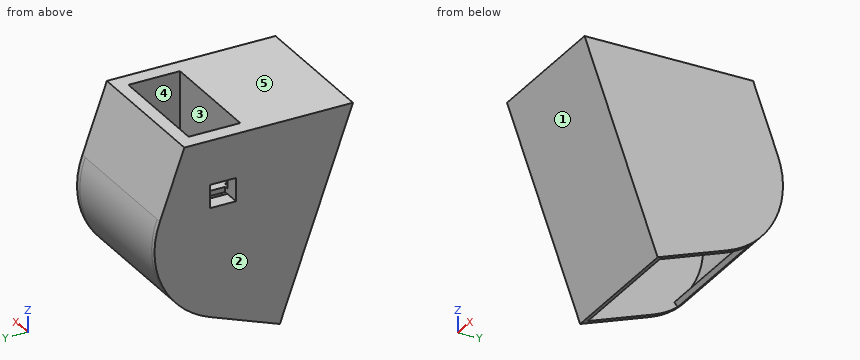
from build123d import *

# Parameters (mm, degrees)
F0_W      = 53.34
F0_H      = 25.4
F0_R      = 1.27
F1_DEPTH  = 2.54
F3_DEPTH  = 53.34
F5_DEPTH  = 7.62
F6_W      = 12.7
F6_H      = 8.89
F7_DEPTH  = 7.62
F8_W      = 12.7
F8_H      = 2.54
F9_DEPTH  = 9.525
F10_W     = 68.58
F10_H     = 41.6090539173
F11_DEPTH = 2.54
F13_REACH = 169.3857709485
F15_DEPTH = 63.5
F17_DEPTH = 2.54
F19_DEPTH = 2.54
F21_DEPTH = 2.54
F22_W     = 63.5
F22_H     = 2.54


with BuildPart() as f1:
    # F0 (on Top) → F1 (new body)
    with BuildSketch(Plane.XY):
        Rectangle(F0_W, F0_H)
        with Locations((-22.86, -8.89)):
            Circle(F0_R, mode=Mode.SUBTRACT)
        with Locations((22.86, -8.89)):
            Circle(F0_R, mode=Mode.SUBTRACT)
        with Locations((-22.86, 8.89)):
            Circle(F0_R, mode=Mode.SUBTRACT)
        with Locations((22.86, 8.89)):
            Circle(F0_R, mode=Mode.SUBTRACT)
    extrude(amount=F1_DEPTH)

    # F2 (on face) → F3 (join, through all)
    with BuildSketch(Plane.YZ.offset(26.67)):
        Polygon((-15.24, -0.447870531), (-9.9437557743, -14.9991819491), (-7.5569365175, -14.130450785), (-12.7, 0), (-12.7, 2.54), (-12.7, 33.02), (-27.4213086776, 33.02), (-26.4968242825, 30.48), (-15.24, 30.48), align=None)
        Polygon((-26.4968242825, 30.48), (-15.24, -0.447870531), (-15.24, 30.48), align=None)
    extrude(amount=-F3_DEPTH)



with BuildPart() as f3:
    # F2 (on face) → F3, piece 2 (new body, through all)
    with BuildSketch(Plane.YZ.offset(26.67)):
        Polygon((12.7, 33.02), (12.7, 30.48), (17.2714728529, 30.48), (28.7046231961, -0.9323224012), (31.0914424529, -0.0635912371), (19.05, 33.02), align=None)
    extrude(amount=-F3_DEPTH)


with BuildPart() as f1_1:
    add(f1.part)

    add(f3.part)  # F5 merges F3
    # F4 (on face) → F5 (join)
    with BuildSketch(Plane.YZ.offset(26.67)):
        Polygon((-27.4213086776, 33.02), (-9.9437557743, -14.9991819491), (31.0914424529, -0.0635912371), (19.05, 33.02), align=None)
    extrude(amount=F5_DEPTH)

    # F6 (on face) → F7 (join)
    with BuildSketch(Plane(origin=(-26.67, 0, 0), x_dir=(0, -1, 0), z_dir=(-1, 0, 0))):
        Polygon((9.9437557743, -14.9991819491), (27.4213086776, 33.02), (-19.05, 33.02), (-31.0914424529, -0.0635912371), align=None)
        with Locations((0, 6.985)):
            Rectangle(F6_W, F6_H, mode=Mode.SUBTRACT)
    extrude(amount=F7_DEPTH)

    # F8 (on face) → F9 (cut)
    with BuildSketch(Plane(origin=(-34.29, 0, 0), x_dir=(0, -1, 0), z_dir=(-1, 0, 0))):
        with Locations((0, 1.27)):
            Rectangle(F8_W, F8_H)
    extrude(amount=-F9_DEPTH, mode=Mode.SUBTRACT)

    # F10 (on face) → F11 (join, through all)
    with BuildSketch(Plane(origin=(0, -13.6012014706, -4.9504324856), x_dir=(1, 0, 0), z_dir=(0, -0.9396926208, -0.3420201433))):
        with Locations((0, -31.4981827789)):
            Rectangle(F10_W, F10_H)
    extrude(amount=-F11_DEPTH)

    f13_end = Plane(origin=(0, -7.2808291762, 33.02), x_dir=(1, 0, 0), z_dir=(0, 0, 1))
    # F12 (on face) → F13 (join, up to a plane its end follows)
    with BuildSketch(Plane(origin=(0, 17.8885802808, -49.1484703875), x_dir=(1, 0, 0), z_dir=(0, 0.3420201433, -0.9396926208))):
        Polygon((31.75, 14.474096284), (34.29, 14.474096284), (34.29, 48.764096284), (-34.29, 48.764096284), (-34.29, 14.474096284), (-31.75, 14.474096284), (-31.75, 46.224096284), (31.75, 46.224096284), align=None)
    f13_long = extrude(amount=-F13_REACH, mode=Mode.PRIVATE)
    add(split(f13_long, bisect_by=f13_end, keep=Keep.BOTTOM, mode=Mode.PRIVATE))

    # F14 (on face) → F15 (join, through all)
    with BuildSketch(Plane(origin=(31.75, 0, 0), x_dir=(0, -1, 0), z_dir=(-1, 0, 0))):
        Polygon((27.4213086775, 33.02), (26.5525775135, 30.6331807432), (60.3402217897, 30.6331807432), (61.2089529537, 33.02), align=None)
    extrude(amount=F15_DEPTH)

    # F16 (on face) → F17 (cut, through all)
    with BuildSketch(Plane(origin=(0, -11.2143822138, -4.0817013215), x_dir=(-1, 0, 0), z_dir=(0, 0.9396926208, 0.3420201433))):
        Polygon((26.67, 4.3436558202), (-26.67, 4.3436558202), (-26.67, -10.6936558203), (-31.75, -10.6936558203), (-31.75, -52.3027097376), (31.75, -52.3027097376), (31.75, -10.6936558203), (26.67, -10.6936558203), align=None)
    extrude(amount=-F17_DEPTH, mode=Mode.SUBTRACT)

    # F18 (on face) → F19 (join)
    with BuildSketch(Plane.YZ.offset(34.29)):
        with BuildLine():
            ThreePointArc((6.6741980668, -53.230171709), (29.9844867323, -31.7454245982), (31.0914424529, -0.0635912371))
            Line((31.0914424529, -0.0635912371), (-7.5569365175, -14.130450785))
            Line((-7.5569365176, -14.130450785), (6.6741980668, -53.230171709))
        make_face()
    extrude(amount=-F19_DEPTH)

    # F20 (on face) → F21 (join)
    with BuildSketch(Plane(origin=(-34.29, 0, 0), x_dir=(0, -1, 0), z_dir=(-1, 0, 0))):
        with BuildLine():
            ThreePointArc((-31.0914424529, -0.0635912371), (-29.9844867323, -31.7454245982), (-6.6741980668, -53.230171709))
            Line((-6.6741980669, -53.230171709), (7.5569365175, -14.130450785))
            Line((7.5569365175, -14.130450785), (-31.0914424529, -0.0635912371))
        make_face()
    extrude(amount=-F21_DEPTH)

    # F24: sweep along a path in F23
    with BuildLine(Plane(origin=(31.75, 0, 0), x_dir=(0, -1, 0), z_dir=(-1, 0, 0))) as f24_path:
        ThreePointArc((-18.5834505022, -46.4695330224), (-32.3206049052, -25.2835298235), (-31.0914424529, -0.0635912371))
    # F22 (on face) → F24 (sweep)
    with BuildSketch(Plane(origin=(0, 3.6574456963, -10.0487494635), x_dir=(1, 0, 0), z_dir=(0, 0.3420201433, -0.9396926208))):
        with Locations((0, -27.9246495586)):
            Rectangle(F22_W, F22_H)
    sweep(path=f24_path.line)


solid = f1_1.part
Geometry check sheet. Reference: the model listing, model coordinates, mm. Face numbers are marked on the shaded views. A direction names the side the tool comes from. Give positions to 0.01 mm unless a question says otherwise; leave off trailing zeros. Loops run counter-clockwise (first coordinate to the right, second up) from the corner with the lowest first, then second, coordinate; pieces in that order, holes last.
(1) Section check C-C on y = 26. Record the cut outline in (x, z).
From the geometry:
outline: (-34.29, -38.59) - (34.29, -38.59) - (34.29, 13.93) - (-34.29, 13.93) - close; hole (-31.75, -33.92) - (31.75, -33.92) - (31.75, -1.92) - (26.67, -1.92) - (26.67, 6.5) - (-26.67, 6.5) - (-26.67, -1.92) - (-31.75, -1.92) - close
(2) Section check A-A on x = 22.86. Record the cut outline in (y, z).
From the geometry:
outline: (-63.91, 33.02) - (-27.93, -65.83) - (-25.55, -64.96) - (-60.34, 30.63) - (-26.55, 30.63) - (-15.09, -0.87) - (-12.7, 0) - (-10.16, 0) - (-10.16, 2.54) - (-12.7, 2.54) - (-12.7, 33.02) - close; (-7.62, 0) - (7.62, 0) - (7.62, 2.54) - (-7.62, 2.54) - close; (10.16, 0) - (12.7, 0) - (12.7, 2.54) - (10.16, 2.54) - close; (12.7, 30.48) - (17.27, 30.48) - (28.7, -0.93) arc R38.59 cw to (17, -44.48) - (18.58, -46.47) arc R41.13 ccw to (31.09, -0.06) - (19.05, 33.02) - (12.7, 33.02) - close
(3) Section check B-B on x = 11. Record the cut outline in (y, z), then the cut area to 3 significant figures.
From the geometry:
outline: (-63.91, 33.02) - (-27.93, -65.83) - (-25.55, -64.96) - (-60.34, 30.63) - (-26.55, 30.63) - (-15.09, -0.87) - (-12.7, 0) - (12.7, 0) - (12.7, 2.54) - (-12.7, 2.54) - (-12.7, 33.02) - close; (12.7, 30.48) - (17.27, 30.48) - (28.7, -0.93) arc R38.59 cw to (17, -44.48) - (18.58, -46.47) arc R41.13 ccw to (31.09, -0.06) - (19.05, 33.02) - (12.7, 33.02) - close
area: 927 mm2
(4) Set-up check for the marked faces 4 and 5: record each of +Z, -Z, +X, -X, +Y, -Y from which the full face is reachable in a straight line by a thin tool's end or side.
From the geometry:
face 4: none
face 5: +Z, +X, -X, +Y, -Y
(5) Release check for a two-part mould opening along Y. For the marked faces 1, 2 and 3 record: released by +Y, released by -Y, zero draft, split by the parting line, or undercut.
From the geometry:
face 1: released by -Y
face 2: zero draft
face 3: undercut
(6) Depth check by flat-ended pin: pin 1 Ø2.5 at (x, y) = (-28.5, -2) entering from -Z; pin 2 Ø2.5 at (x, y) = (-10.5, 14) entering from -Z; pin 3 Ø3 at (x, z) = (7, 31) entering from -Y. Enter the tip coordinate at first touch or a pass-through.
From the geometry:
pin 1: stops at z = -12.56
pin 2: stops at z = 30.48
pin 3: stops at y = -63.72
(7) Thickness scan on L1, parallel to Y at x = 22.86, z = 1.8; L2, parallel to Y at x = 22.86, z = 0.7; L3, parallel to X at y = -20.5, z = -37.5. Record the ranges inside material, lowest first.
From the geometry:
L1: y = -52.55 to -49.85, -16.06 to -10.16, -7.62 to 7.62, 10.16 to 12.7, 27.71 to 30.41
L2: y = -52.15 to -49.45, -15.66 to -10.16, -7.62 to 7.62, 10.16 to 12.7, 28.11 to 30.81
L3: x = -34.29 to -31.75, 31.75 to 34.29
(8) Section check D-D on z = 23.5. Record the cut outline in (x, y) (3 decimals), then the cut area to 3 significant figures.
From the geometry:
outline: (-34.29, -60.447) - (34.29, -60.447) - (34.29, 22.515) - (-34.29, 22.515) - close; hole (-31.75, -57.744) - (31.75, -57.744) - (31.75, -23.956) - (-31.75, -23.956) - close; hole (-26.67, -12.7) - (26.67, -12.7) - (26.67, 19.812) - (-26.67, 19.812) - close
area: 1,810 mm2
